The model under review builds one solid part; all positions refer to its coordinate system, in mm. A direction names the side the tool comes from. Give positions to 0.01 mm unless a question says otherwise; leave off trailing zeros. Loops run counter-clockwise (first coordinate to the right, second up) from the corner with the lowest first, then second, coordinate; pieces in that order, holes last. Notation, with made-up numbers: M 28,-14 L 86,-14 A10 ccw 86,4 Z; hole C -36,41 d8. An arc over 180 degrees is marked long. One line per item, written item: value. Start each with the question number.
Q1. For pin 1 (6 mm diameter, centred on x = 5, z = -1.5, fed in from +Y); pin 2 (0.8 mm diameter, centred on y = -1, z = 7, fed in from +X); pin 3 (0.8 mm diameter, centred on y = -2, z = 7, fed in from -X), all flat-tipped, find the tip position at first contact; note any pin that passes through.
Q2. Mouldability with a two-part tool opening along Z and no side actions: class faces 1 (the face through (-18.701, -1.479, -1.215)), 2 (the face through (-1.79, -1.48, 12.2)), 3 (the face through (21, -1, -12.496)), 4 (the face through (-19.002, -1, 0)) as released by +Z, released by -Z, zero draft, split by the parting line, or undercut.
Q3. We need section B-B on z = -4.5. Write out the cut boundary in (x, y), plus the area to 3 significant figures.
Q4. For faces 5 (the face through (0, -3, 3)), 6 (the face through (11.287, -1.479, -5.796)), 7 (the face through (-6.7, -1.48, -8.21)), list the 3-axis set-ups (+Z, -Z, +X, -X, +Y, -Y) from which the entire face can be reached by the end or side of a thin tool; tool diameter is ignored.
Q5. We need section A-A on z = -10.5. Write out the cut boundary in (x, y), plus the area to 3 significant figures.
Q6. To check wall thickness, follow line 1 along Z through (x, y) = (16, -0.2); line 2 along Z through (x, y) = (-25.5, -1.55); line 3 along X through (y, z) = (-0.6, 11.25). State the ranges of each line that lie inside material, in increasing order. Write a range as from..to.
```python
from build123d import *

# Parameters (mm, degrees)
F1_DEPTH = 3


# Not quite as in the source:
# - a feature names something its author has since deleted; it is built from what else it names


with BuildPart() as f1:
    # F0 (on Front) → F1 (new body)
    with BuildSketch(Plane.XZ):
        with BuildLine():
            Line((-23.0000003952, 0), (-19.0015753579, 0))
            Line((-19.0015753579, 0), (-19.0015753579, 0.5))
            ThreePointArc((-19.0015753579, 0.5), (-18.7086821391, 1.2071067812), (-18.0015753579, 1.5))
            Line((-18.0015753579, 1.5), (-2, 1.5))
            ThreePointArc((-2, 1.5), (-1.1180339887, 2.2360679775), (0, 2.5))
            Line((0, 2.5), (0, 5.4957361976))
            Line((0, 5.4957361976), (-6.0015753579, 5.4957361976))
            ThreePointArc((-6.0015753579, 5.4957361976), (-6.7086821391, 5.7886294164), (-7.0015753579, 6.4957361976))
            Line((-7.0015753579, 6.4957361976), (-7.0015753579, 7.4957361976))
            ThreePointArc((-7.0015753579, 7.4957361976), (-6.7086821391, 8.2028429788), (-6.0015753579, 8.4957361976))
            Line((-6.0015753579, 8.4957361976), (-2.5015753579, 8.4957361976))
            ThreePointArc((-2.5015753579, 8.4957361976), (-1.7944685767, 8.7886294164), (-1.5015753579, 9.4957361976))
            Line((-1.5015753579, 9.4957361976), (-1.5015753579, 11.4957361976))
            ThreePointArc((-1.5015753579, 11.4957361976), (-1.7944685767, 12.2028429788), (-2.5015753579, 12.4957361976))
            Line((-2.5015753579, 12.4957361976), (-10.0015753579, 12.4957361976))
            ThreePointArc((-10.0015753579, 12.4957361976), (-10.7086821391, 12.2028429788), (-11.0015753579, 11.4957361976))
            Line((-11.0015753579, 11.4957361976), (-11.0015753579, 8.4957361976))
            Line((-11.0015753579, 8.4957361976), (-11.0015753579, 6.4957361976))
            ThreePointArc((-11.0015753579, 6.4957361976), (-11.2944685767, 5.7886294164), (-12.0015753579, 5.4957361976))
            Line((-12.0015753579, 5.4957361976), (-18.0015753579, 5.4957361976))
            ThreePointArc((-18.0015753579, 5.4957361976), (-18.7086821391, 5.7886294164), (-19.0015753579, 6.4957361976))
            Line((-19.0015753579, 6.4957361976), (-19.0015753579, 7.4957361976))
            ThreePointArc((-19.0015753579, 7.4957361976), (-18.7086821391, 8.2028429788), (-18.0015753579, 8.4957361976))
            Line((-18.0015753579, 8.4957361976), (-15.0015753579, 8.4957361976))
            ThreePointArc((-15.0015753579, 8.4957361976), (-14.2944685767, 8.7886294164), (-14.0015753579, 9.4957361976))
            Line((-14.0015753579, 9.4957361976), (-14.0015753579, 11.4957361976))
            ThreePointArc((-14.0015753579, 11.4957361976), (-14.2944685767, 12.2028429788), (-15.0015753579, 12.4957361976))
            Line((-15.0015753579, 12.4957361976), (-28.0015753579, 12.4957361976))
            ThreePointArc((-28.0015753579, 12.4957361976), (-28.7086821391, 12.2028429788), (-29.0015753579, 11.4957361976))
            Line((-29.0015753579, 11.4957361976), (-29.0015753579, 9.4957361976))
            ThreePointArc((-29.0015753579, 9.4957361976), (-28.7086821391, 8.7886294164), (-28.0015753579, 8.4957361976))
            Line((-28.0015753579, 8.4957361976), (-24.0015753579, 8.4957361976))
            ThreePointArc((-24.0015753579, 8.4957361976), (-23.294403037, 8.2028542282), (-23.0013899752, 7.4957362148))
            Line((-23.0013899752, 7.4957362148), (-23.0000003952, 0))
        make_face()
        with BuildLine():
            Line((19.0015753579, 0.5), (19.0015753579, 0))
            Line((19.0015753579, 0), (23.0000003952, 0))
            Line((23.0000003952, 0), (23.0013899752, 7.4957362148))
            ThreePointArc((23.0013899752, 7.4957362148), (23.294403037, 8.2028542282), (24.0015753579, 8.4957361976))
            Line((24.0015753579, 8.4957361976), (28.0015753579, 8.4957361976))
            ThreePointArc((28.0015753579, 8.4957361976), (28.7086821391, 8.7886294164), (29.0015753579, 9.4957361976))
            Line((29.0015753579, 9.4957361976), (29.0015753579, 11.4957361976))
            ThreePointArc((29.0015753579, 11.4957361976), (28.7086821391, 12.2028429788), (28.0015753579, 12.4957361976))
            Line((28.0015753579, 12.4957361976), (15.0015753579, 12.4957361976))
            ThreePointArc((15.0015753579, 12.4957361976), (14.2944685767, 12.2028429788), (14.0015753579, 11.4957361976))
            Line((14.0015753579, 11.4957361976), (14.0015753579, 9.4957361976))
            ThreePointArc((14.0015753579, 9.4957361976), (14.2944685767, 8.7886294164), (15.0015753579, 8.4957361976))
            Line((15.0015753579, 8.4957361976), (18.0015753579, 8.4957361976))
            ThreePointArc((18.0015753579, 8.4957361976), (18.7086821391, 8.2028429788), (19.0015753579, 7.4957361976))
            Line((19.0015753579, 7.4957361976), (19.0015753579, 6.4957361976))
            ThreePointArc((19.0015753579, 6.4957361976), (18.7086821391, 5.7886294164), (18.0015753579, 5.4957361976))
            Line((18.0015753579, 5.4957361976), (12.0015753579, 5.4957361976))
            ThreePointArc((12.0015753579, 5.4957361976), (11.2944685767, 5.7886294164), (11.0015753579, 6.4957361976))
            Line((11.0015753579, 6.4957361976), (11.0015753579, 8.4957361976))
            Line((11.0015753579, 8.4957361976), (11.0015753579, 11.4957361976))
            ThreePointArc((11.0015753579, 11.4957361976), (10.7086821391, 12.2028429788), (10.0015753579, 12.4957361976))
            Line((10.0015753579, 12.4957361976), (2.5015753579, 12.4957361976))
            ThreePointArc((2.5015753579, 12.4957361976), (1.7944685767, 12.2028429788), (1.5015753579, 11.4957361976))
            Line((1.5015753579, 11.4957361976), (1.5015753579, 9.4957361976))
            ThreePointArc((1.5015753579, 9.4957361976), (1.7944685767, 8.7886294164), (2.5015753579, 8.4957361976))
            Line((2.5015753579, 8.4957361976), (6.0015753579, 8.4957361976))
            ThreePointArc((6.0015753579, 8.4957361976), (6.7086821391, 8.2028429788), (7.0015753579, 7.4957361976))
            Line((7.0015753579, 7.4957361976), (7.0015753579, 6.4957361976))
            ThreePointArc((7.0015753579, 6.4957361976), (6.7086821391, 5.7886294164), (6.0015753579, 5.4957361976))
            Line((6.0015753579, 5.4957361976), (0, 5.4957361976))
            Line((0, 5.4957361976), (0, 2.5))
            ThreePointArc((0, 2.5), (1.1180339887, 2.2360679775), (2, 1.5))
            Line((2, 1.5), (18.0015753579, 1.5))
            ThreePointArc((18.0015753579, 1.5), (18.7086821391, 1.2071067812), (19.0015753579, 0.5))
        make_face()
        with BuildLine():
            Line((-6.0015753579, -5.4957361976), (0, -5.4957361976))
            Line((0, -5.4957361976), (0, -2.5))
            ThreePointArc((0, -2.5), (-1.1180339887, -2.2360679775), (-2, -1.5))
            Line((-2, -1.5), (-18.0015753579, -1.5))
            ThreePointArc((-18.0015753579, -1.5), (-18.7086821391, -1.2071067812), (-19.0015753579, -0.5))
            Line((-19.0015753579, -0.5), (-19.0015753579, 0))
            Line((-19.0015753579, 0), (-23.0000003952, 0))
            Line((-23.0000003952, 0), (-23.0013899752, -7.4957362148))
            ThreePointArc((-23.0013899752, -7.4957362148), (-23.294403037, -8.2028542282), (-24.0015753579, -8.4957361976))
            Line((-24.0015753579, -8.4957361976), (-28.0015753579, -8.4957361976))
            ThreePointArc((-28.0015753579, -8.4957361976), (-28.7086821391, -8.7886294164), (-29.0015753579, -9.4957361976))
            Line((-29.0015753579, -9.4957361976), (-29.0015753579, -11.4957361976))
            ThreePointArc((-29.0015753579, -11.4957361976), (-28.7086821391, -12.2028429788), (-28.0015753579, -12.4957361976))
            Line((-28.0015753579, -12.4957361976), (-15.0015753579, -12.4957361976))
            ThreePointArc((-15.0015753579, -12.4957361976), (-14.2944685767, -12.2028429788), (-14.0015753579, -11.4957361976))
            Line((-14.0015753579, -11.4957361976), (-14.0015753579, -9.4957361976))
            ThreePointArc((-14.0015753579, -9.4957361976), (-14.2944685767, -8.7886294164), (-15.0015753579, -8.4957361976))
            Line((-15.0015753579, -8.4957361976), (-18.0015753579, -8.4957361976))
            ThreePointArc((-18.0015753579, -8.4957361976), (-18.7086821391, -8.2028429788), (-19.0015753579, -7.4957361976))
            Line((-19.0015753579, -7.4957361976), (-19.0015753579, -6.4957361976))
            ThreePointArc((-19.0015753579, -6.4957361976), (-18.7086821391, -5.7886294164), (-18.0015753579, -5.4957361976))
            Line((-18.0015753579, -5.4957361976), (-12.0015753579, -5.4957361976))
            ThreePointArc((-12.0015753579, -5.4957361976), (-11.2944685767, -5.7886294164), (-11.0015753579, -6.4957361976))
            Line((-11.0015753579, -6.4957361976), (-11.0015753579, -8.4957361976))
            Line((-11.0015753579, -8.4957361976), (-11.0015753579, -11.4957361976))
            ThreePointArc((-11.0015753579, -11.4957361976), (-10.7086821391, -12.2028429788), (-10.0015753579, -12.4957361976))
            Line((-10.0015753579, -12.4957361976), (-2.5015753579, -12.4957361976))
            ThreePointArc((-2.5015753579, -12.4957361976), (-1.7944685767, -12.2028429788), (-1.5015753579, -11.4957361976))
            Line((-1.5015753579, -11.4957361976), (-1.5015753579, -9.4957361976))
            ThreePointArc((-1.5015753579, -9.4957361976), (-1.7944685767, -8.7886294164), (-2.5015753579, -8.4957361976))
            Line((-2.5015753579, -8.4957361976), (-6.0015753579, -8.4957361976))
            ThreePointArc((-6.0015753579, -8.4957361976), (-6.7086821391, -8.2028429788), (-7.0015753579, -7.4957361976))
            Line((-7.0015753579, -7.4957361976), (-7.0015753579, -6.4957361976))
            ThreePointArc((-7.0015753579, -6.4957361976), (-6.7086821391, -5.7886294164), (-6.0015753579, -5.4957361976))
        make_face()
        with BuildLine():
            ThreePointArc((1.5015753579, -11.4957361976), (1.7944685767, -12.2028429788), (2.5015753579, -12.4957361976))
            Line((2.5015753579, -12.4957361976), (10.0015753579, -12.4957361976))
            ThreePointArc((10.0015753579, -12.4957361976), (10.7086821391, -12.2028429788), (11.0015753579, -11.4957361976))
            Line((11.0015753579, -11.4957361976), (11.0015753579, -8.4957361976))
            Line((11.0015753579, -8.4957361976), (11.0015753579, -6.4957361976))
            ThreePointArc((11.0015753579, -6.4957361976), (11.2944685767, -5.7886294164), (12.0015753579, -5.4957361976))
            Line((12.0015753579, -5.4957361976), (18.0015753579, -5.4957361976))
            ThreePointArc((18.0015753579, -5.4957361976), (18.7086821391, -5.7886294164), (19.0015753579, -6.4957361976))
            Line((19.0015753579, -6.4957361976), (19.0015753579, -7.4957361976))
            ThreePointArc((19.0015753579, -7.4957361976), (18.7086821391, -8.2028429788), (18.0015753579, -8.4957361976))
            Line((18.0015753579, -8.4957361976), (15.0015753579, -8.4957361976))
            ThreePointArc((15.0015753579, -8.4957361976), (14.2944685767, -8.7886294164), (14.0015753579, -9.4957361976))
            Line((14.0015753579, -9.4957361976), (14.0015753579, -11.4957361976))
            ThreePointArc((14.0015753579, -11.4957361976), (14.2944685767, -12.2028429788), (15.0015753579, -12.4957361976))
            Line((15.0015753579, -12.4957361976), (28.0015753579, -12.4957361976))
            ThreePointArc((28.0015753579, -12.4957361976), (28.7086821391, -12.2028429788), (29.0015753579, -11.4957361976))
            Line((29.0015753579, -11.4957361976), (29.0015753579, -9.4957361976))
            ThreePointArc((29.0015753579, -9.4957361976), (28.7086821391, -8.7886294164), (28.0015753579, -8.4957361976))
            Line((28.0015753579, -8.4957361976), (24.0015753579, -8.4957361976))
            ThreePointArc((24.0015753579, -8.4957361976), (23.294403037, -8.2028542282), (23.0013899752, -7.4957362148))
            Line((23.0013899752, -7.4957362148), (23.0000003952, 0))
            Line((23.0000003952, 0), (19.0015753579, 0))
            Line((19.0015753579, 0), (19.0015753579, -0.5))
            ThreePointArc((19.0015753579, -0.5), (18.7086821391, -1.2071067812), (18.0015753579, -1.5))
            Line((18.0015753579, -1.5), (2, -1.5))
            ThreePointArc((2, -1.5), (1.1180339887, -2.2360679775), (0, -2.5))
            Line((0, -2.5), (0, -5.4957361976))
            Line((0, -5.4957361976), (6.0015753579, -5.4957361976))
            ThreePointArc((6.0015753579, -5.4957361976), (6.7086821391, -5.7886294164), (7.0015753579, -6.4957361976))
            Line((7.0015753579, -6.4957361976), (7.0015753579, -7.4957361976))
            ThreePointArc((7.0015753579, -7.4957361976), (6.7086821391, -8.2028429788), (6.0015753579, -8.4957361976))
            Line((6.0015753579, -8.4957361976), (2.5015753579, -8.4957361976))
            ThreePointArc((2.5015753579, -8.4957361976), (1.7944685767, -8.7886294164), (1.5015753579, -9.4957361976))
            Line((1.5015753579, -9.4957361976), (1.5015753579, -11.4957361976))
        make_face()
    extrude(amount=F1_DEPTH)


solid = f1.part
```
Solved:
1. pin 1: y = 0
1. pin 2: x = 23
1. pin 3: x = -23
2. face 1: undercut
2. face 2: released by +Z
2. face 3: released by -Z
2. face 4: undercut
3. outline: M -23,-3 L 23,-3 L 23,0 L -23,0 Z
3. area: 138 mm2
4. face 5: +Z, -Z, +X, -X, -Y
4. face 6: -Z, +Y, -Y
4. face 7: +Y, -Y
5. outline: M -29,-3 L -14,-3 L -14,0 L -29,0 Z; M -11,-3 L -1.5,-3 L -1.5,0 L -11,0 Z; M 1.5,-3 L 11,-3 L 11,0 L 1.5,0 Z; M 14,-3 L 29,-3 L 29,0 L 14,0 Z
5. area: 147 mm2
6. line 1: -12.5..-8.5, -5.5..-1.5, 1.5..5.5, 8.5..12.5
6. line 2: -12.5..-8.5, 8.5..12.5
6. line 3: -29..-14, -11..-1.5, 1.5..11, 14..29
